Verification items for the finished model (mm, model axes). Coordinates: 2 decimals unless noted, no trailing zeros. Order: outer loops, then holes, each group sorted by start corner. A loop starts at its lowest first (then second) coordinate and runs counter-clockwise, first axis right, second up. Notation, with made-up numbers: M 44,-36 L 67,-36 A23 cw 67,-1 Z; hole C 13,-37.75 d7. An arc over 180 degrees is marked long. Return JSON: item names as keys, results as strings.
```python
from build123d import *

# Parameters (mm, degrees)
SKETCH1_R           = 2.75
BOSS_EXTRUDE1_DEPTH = 6.35
SKETCH4_W           = 27.5
SKETCH4_H           = 6
BOSS_EXTRUDE2_DEPTH = 6.35
CUT_EXTRUDE1_DEPTH  = 6.35
CUT_EXTRUDE2_DEPTH  = 1
FILLET1_R           = 2
SKETCH5_R           = 2.25
SKETCH5_R_2         = 1.75
SKETCH5_R_3         = 2.1
CUT_EXTRUDE3_DEPTH  = 329.865964338


with BuildPart() as part:
    # Sketch1 → Boss-Extrude1 (new body)
    with BuildSketch(Plane.XY):
        Polygon((182, -212), (212, -212), (212, -182), (232.5, -182), (232.5, 0), (232.5, 182), (212, 182), (212, 212), (182, 212), (182, 232.5), (17.5, 232.5), (17.5, 186.5), (-45.5, 186.5), (-45.5, 232.5), (-182, 232.5), (-182, 212), (-212, 212), (-212, 182), (-232.5, 182), (-232.5, 0), (-232.5, -182), (-212, -182), (-212, -212), (-182, -212), (-182, -232.5), (-17.5, -232.5), (-17.5, -186.5), (45.5, -186.5), (45.5, -232.5), (182, -232.5), align=None)
        with Locations((-222.5, -162)):
            Circle(SKETCH1_R, mode=Mode.SUBTRACT)
        with Locations(Location((222.5, -162, 0), (0, 0, 180))):
            Circle(SKETCH1_R, mode=Mode.SUBTRACT)
        with Locations((222.5, 162)):
            Circle(SKETCH1_R, mode=Mode.SUBTRACT)
        with Locations(Location((-222.5, 162, 0), (0, 0, 180))):
            Circle(SKETCH1_R, mode=Mode.SUBTRACT)
        with Locations((-222.5, 0)):
            Circle(SKETCH1_R, mode=Mode.SUBTRACT)
        with Locations((222.5, 0)):
            Circle(SKETCH1_R, mode=Mode.SUBTRACT)
        with Locations((-113.75, 222.5)):
            Circle(SKETCH1_R, mode=Mode.SUBTRACT)
        with Locations((99.75, 222.5)):
            Circle(SKETCH1_R, mode=Mode.SUBTRACT)
        with Locations(Location((99.75, -222.5, 0), (0, 0, 180))):
            Circle(SKETCH1_R, mode=Mode.SUBTRACT)
        with Locations(Location((-113.75, -222.5, 0), (0, 0, 180))):
            Circle(SKETCH1_R, mode=Mode.SUBTRACT)
    extrude(amount=BOSS_EXTRUDE1_DEPTH)

    # Sketch4 → Boss-Extrude2 (add)
    with BuildSketch(Plane.XY.offset(6.35)):
        with Locations((31.75, -189.5)):
            Rectangle(SKETCH4_W, SKETCH4_H)
        with Locations((-31.75, 189.5)):
            Rectangle(SKETCH4_W, SKETCH4_H)
    extrude(amount=-BOSS_EXTRUDE2_DEPTH)

    # Sketch2 → Cut-Extrude1 (cut)
    with BuildSketch(Plane.XY.offset(6.35)):
        with BuildLine():
            Line((212, 212), (182, 212))
            ThreePointArc((182, 212), (190.786796564, 190.786796564), (212, 182))
            Line((212, 182), (212, 212))
        make_face()
        with BuildLine():
            Line((182, -212), (212, -212))
            Line((212, -212), (212, -182))
            ThreePointArc((212, -182), (190.786796564, -190.786796564), (182, -212))
        make_face()
        with BuildLine():
            Line((-212, -212), (-182, -212))
            ThreePointArc((-182, -212), (-190.786796564, -190.786796564), (-212, -182))
            Line((-212, -182), (-212, -212))
        make_face()
        with BuildLine():
            Line((-212, 212), (-212, 182))
            ThreePointArc((-212, 182), (-190.786796564, 190.786796564), (-182, 212))
            Line((-182, 212), (-212, 212))
        make_face()
    extrude(amount=-CUT_EXTRUDE1_DEPTH, mode=Mode.SUBTRACT)

    # Sketch3 → Cut-Extrude2 (cut)
    with BuildSketch(Plane.XY.offset(6.35)):
        with BuildLine():
            Line((-90.71398693, 34.138368447), (-32.791230158, 10.145977022))
            ThreePointArc((-32.791230158, 10.145977022), (34.325, 0), (-32.791230158, -10.145977022))
            Line((-32.791230158, -10.145977022), (-90.71398693, -34.138368447))
            ThreePointArc((-90.71398693, -34.138368447), (-88.022539954, -40.576940312), (-84.874800654, -46.805168935))
            Line((-84.874800654, -46.805168935), (-103.008511577, -76.276321146))
            ThreePointArc((-103.008511577, -76.276321146), (-90.633411679, -90.633411679), (-76.276321146, -103.008511577))
            Line((-76.276321146, -103.008511577), (-46.805168935, -84.874800654))
            ThreePointArc((-46.805168935, -84.874800654), (-37.091591682, -89.547023689), (-26.919294746, -93.111799442))
            Line((-26.919294746, -93.111799442), (-18.90251313, -126.773520983))
            ThreePointArc((-18.90251313, -126.773520983), (0, -128.175), (18.90251313, -126.773520983))
            Line((18.90251313, -126.773520983), (26.919294746, -93.111799442))
            ThreePointArc((26.919294746, -93.111799442), (37.091591682, -89.547023689), (46.805168935, -84.874800654))
            Line((46.805168935, -84.874800654), (76.276321146, -103.008511577))
            ThreePointArc((76.276321146, -103.008511577), (90.633411679, -90.633411679), (103.008511577, -76.276321146))
            Line((103.008511577, -76.276321146), (84.874800654, -46.805168935))
            ThreePointArc((84.874800654, -46.805168935), (89.547023689, -37.091591682), (93.111799442, -26.919294746))
            Line((93.111799442, -26.919294746), (126.773520983, -18.90251313))
            ThreePointArc((126.773520983, -18.90251313), (128.175, 0), (126.773520983, 18.90251313))
            Line((126.773520983, 18.90251313), (93.111799442, 26.919294746))
            ThreePointArc((93.111799442, 26.919294746), (89.547023689, 37.091591682), (84.874800654, 46.805168935))
            Line((84.874800654, 46.805168935), (103.008511577, 76.276321146))
            ThreePointArc((103.008511577, 76.276321146), (90.633411679, 90.633411679), (76.276321146, 103.008511577))
            Line((76.276321146, 103.008511577), (46.805168935, 84.874800654))
            ThreePointArc((46.805168935, 84.874800654), (37.091591682, 89.547023689), (26.919294746, 93.111799442))
            Line((26.919294746, 93.111799442), (18.90251313, 126.773520983))
            ThreePointArc((18.90251313, 126.773520983), (0, 128.175), (-18.90251313, 126.773520983))
            Line((-18.90251313, 126.773520983), (-26.919294746, 93.111799442))
            ThreePointArc((-26.919294746, 93.111799442), (-37.091591682, 89.547023689), (-46.805168935, 84.874800654))
            Line((-46.805168935, 84.874800654), (-76.276321146, 103.008511577))
            ThreePointArc((-76.276321146, 103.008511577), (-90.633411679, 90.633411679), (-103.008511577, 76.276321146))
            Line((-103.008511577, 76.276321146), (-84.874800654, 46.805168935))
            ThreePointArc((-84.874800654, 46.805168935), (-88.022539954, 40.576940312), (-90.71398693, 34.138368447))
        make_face()
        with BuildLine():
            Line((-82.41394096, 37.57356731), (-36.249121046, 18.451472797))
            ThreePointArc((-36.249121046, 18.451472797), (40.675, 0), (-36.249121046, -18.451472797))
            Line((-36.249121046, -18.451472797), (-82.41394096, -37.57356731))
            ThreePointArc((-82.41394096, -37.57356731), (-80.084171036, -42.312600659), (-77.482180911, -46.907806027))
            Line((-77.482180911, -46.907806027), (-95.308362806, -75.879157904))
            ThreePointArc((-95.308362806, -75.879157904), (-86.143283618, -86.143283618), (-75.879157904, -95.308362806))
            Line((-75.879157904, -95.308362806), (-46.907806027, -77.482180911))
            ThreePointArc((-46.907806027, -77.482180911), (-34.661551886, -83.680388657), (-21.619347811, -87.957003276))
            Line((-21.619347811, -87.957003276), (-13.73852254, -121.047856749))
            ThreePointArc((-13.73852254, -121.047856749), (0, -121.825), (13.73852254, -121.047856749))
            Line((13.73852254, -121.047856749), (21.619347811, -87.957003276))
            ThreePointArc((21.619347811, -87.957003276), (34.661551886, -83.680388657), (46.907806027, -77.482180911))
            Line((46.907806027, -77.482180911), (75.879157904, -95.308362806))
            ThreePointArc((75.879157904, -95.308362806), (86.143283618, -86.143283618), (95.308362806, -75.879157904))
            Line((95.308362806, -75.879157904), (77.482180911, -46.907806027))
            ThreePointArc((77.482180911, -46.907806027), (83.680388657, -34.661551886), (87.957003276, -21.619347811))
            Line((87.957003276, -21.619347811), (121.047856749, -13.73852254))
            ThreePointArc((121.047856749, -13.73852254), (121.825, 0), (121.047856749, 13.73852254))
            Line((121.047856749, 13.73852254), (87.957003276, 21.619347811))
            ThreePointArc((87.957003276, 21.619347811), (83.680388657, 34.661551886), (77.482180911, 46.907806027))
            Line((77.482180911, 46.907806027), (95.308362806, 75.879157904))
            ThreePointArc((95.308362806, 75.879157904), (86.143283618, 86.143283618), (75.879157904, 95.308362806))
            Line((75.879157904, 95.308362806), (46.907806027, 77.482180911))
            ThreePointArc((46.907806027, 77.482180911), (34.661551886, 83.680388657), (21.619347811, 87.957003276))
            Line((21.619347811, 87.957003276), (13.73852254, 121.047856749))
            ThreePointArc((13.73852254, 121.047856749), (0, 121.825), (-13.73852254, 121.047856749))
            Line((-13.73852254, 121.047856749), (-21.619347811, 87.957003276))
            ThreePointArc((-21.619347811, 87.957003276), (-34.661551886, 83.680388657), (-46.907806027, 77.482180911))
            Line((-46.907806027, 77.482180911), (-75.879157904, 95.308362806))
            ThreePointArc((-75.879157904, 95.308362806), (-86.143283618, 86.143283618), (-95.308362806, 75.879157904))
            Line((-95.308362806, 75.879157904), (-77.482180911, 46.907806027))
            ThreePointArc((-77.482180911, 46.907806027), (-80.084171036, 42.312600659), (-82.41394096, 37.57356731))
        make_face(mode=Mode.SUBTRACT)
    extrude(amount=-CUT_EXTRUDE2_DEPTH, mode=Mode.SUBTRACT)

    # Fillet1
    fillet1_edges = [part.edges().sort_by_distance(p)[0] for p in [
        (45.5, -192.5, 3.175),
        (18, -192.5, 3.175),
        (18, -186.5, 3.175),
        (-45.5, 192.5, 3.175),
        (-18, 192.5, 3.175),
        (-18, 186.5, 3.175),
        (17.5, 186.5, 3.175),
        (-17.5, -186.5, 3.175),
    ]]
    fillet(fillet1_edges, radius=FILLET1_R)

    # Sketch5 → Cut-Extrude3 (cut, through all)
    with BuildSketch(Plane(origin=(0, 0, 0), x_dir=(-1, 0, 0), z_dir=(0, 0, -1))):
        with Locations((-129.75, 119)):
            Circle(SKETCH5_R)
        with Locations((57.83, -137.299993563)):
            Circle(SKETCH5_R_2)
        with Locations((178.5, -136.299993563)):
            Circle(SKETCH5_R_2)
        with Locations((-178.25, 119)):
            Circle(SKETCH5_R)
        with Locations((178.5, -182.499993563)):
            Circle(SKETCH5_R_2)
        with Locations((57.83, -181.499993563)):
            Circle(SKETCH5_R_2)
        with Locations((-170, 50)):
            Circle(SKETCH5_R_3)
        with Locations((-120, 50)):
            Circle(SKETCH5_R_3)
        with Locations((-170, -100)):
            Circle(SKETCH5_R_3)
        with Locations((-120, -100)):
            Circle(SKETCH5_R_3)
    extrude(amount=-CUT_EXTRUDE3_DEPTH, mode=Mode.SUBTRACT)


solid = part.part
```
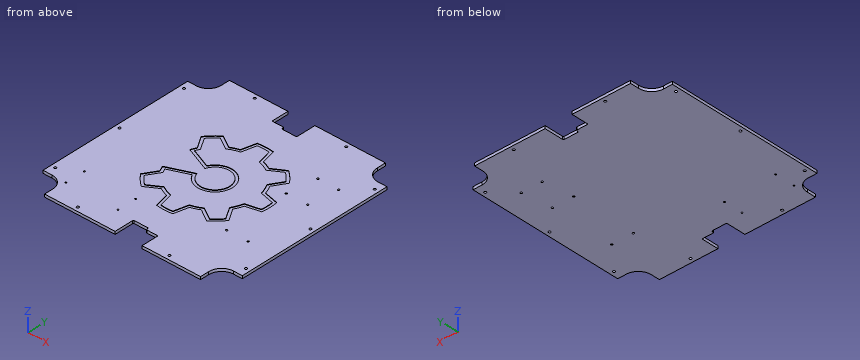
Q1. Cross-section at A-A, the plane x = 0. Record the boundary of the cut face in (y, z) (3 decimals), and give its area (3 significant figures).
Values:
{"outline": "M -186.5,0 L 186.5,0 L 186.5,6.35 L 128.175,6.35 L 128.175,5.35 L 121.825,5.35 L 121.825,6.35 L 40.675,6.35 L 40.675,5.35 L 34.325,5.35 L 34.325,6.35 L -34.325,6.35 L -34.325,5.35 L -40.675,5.35 L -40.675,6.35 L -121.825,6.35 L -121.825,5.35 L -128.175,5.35 L -128.175,6.35 L -186.5,6.35 Z", "area": "2,340 mm^2"}
Q2. Go/stop test with flat-tipped pins: pin 1 (5 mm diameter, centred on x = 222.5, y = 162, fed in from +Z); pin 2 (3 mm diameter, centred on y = -203, z = 2, fed in from +X); pin 3 (1.9 mm diameter, centred on y = -218.5, z = 4, fed in from -X); pin 4 (1.9 mm diameter, centred on x = 2, z = 4.5, fed in from +Y). Record where each tip stops, or that it passes through.
Values:
{"pin 1": "through", "pin 2": "x = 183.9", "pin 3": "x = -182", "pin 4": "y = 186.5"}
Q3. Material ranges on line 1 along Y through (x, z) = (222.5, 1.5); line 2 along X through (y, z) = (-162, 2.25), recorded low to high.
Values:
{"line 1": "-182 to -164.75, -159.25 to -2.75, 2.75 to 159.25, 164.75 to 182", "line 2": "-232.5 to -225.25, -219.75 to 219.75, 225.25 to 232.5"}
Q4. Cross-section at B-B, the plane z = 3.5. State how many separate pieces and enclosed holes the cut face has, and give its area (3 significant figures).
Values:
{"separate pieces": "1", "enclosed holes": "20", "area": "201,000 mm^2"}
